Autodesk Inventor part; units mm, degrees
ref_plane "YZ Plane" through (0, 0, 0) normal (1, 0, 0) x (0, 1, 0)
ref_plane "XZ Plane" through (0, 0, 0) normal (0, 1, 0) x (-1, 0, 0)
ref_plane "XY Plane" through (0, 0, 0) normal (0, 0, 1) x (1, 0, 0)
sketch "Esquisse1" plane through (0, 0, 0) normal (0, 1, 0) x (-1, 0, 0)
  line L0 (20.5, 10.5) -> (-20.5, 10.5)
  line L1 (-20.5, 10.5) -> (-20.5, -10.5)
  line L2 (-20.5, -10.5) -> (20.5, -10.5)
  line L3 (20.5, -10.5) -> (20.5, 10.5)
  line L4 (28.5, 12.5) -> (-36.5, 12.5)
  line L5 (-36.5, 12.5) -> (-36.5, -12.5)
  line L6 (-36.5, -12.5) -> (28.5, -12.5)
  line L7 (28.5, -12.5) -> (28.5, 12.5)
  line L8 (-36.5, -12.5) -> (-45.5993, 12.5)
  line L9 (-45.5993, 12.5) -> (-36.5, 12.5)
  point P0 (0, 0)
  dimension "d0" = 20
  dimension "d1" = 41
  dimension "d2" = 21
  dimension "d3" = 10.5
  dimension "d4" = 20.5
  dimension "d5" = 8
  dimension "d6" = 2
  dimension "d7" = 2
  dimension "d8" = 16
extrude "Extrusion1" add sketch "Esquisse1" along normal mid plane 25
sketch "Esquisse2" plane through (36.5, -12.5, -12.5) normal (0.9397, 0, -0.342) x (-0.342, 0, -0.9397)
  line L0 (-26.6044, 25) -> (0, 0)
  line L1 (0, 0) -> (0, 25)
  line L2 (0, 25) -> (-26.6044, 0)
  arc A0 (-8.3022, 22.298) -> (-18.3022, 22.298) centre (-13.3022, 12.5) ccw
  line L3 (-18.3022, 22.298) -> (-8.3022, 22.298)
  line L4 (-8.3022, 22.298) -> (-8.3022, 2.702)
  line L5 (-8.3022, 2.702) -> (-18.3022, 2.702)
  line L6 (-18.3022, 2.702) -> (-18.3022, 22.298)
  arc A1 (-8.3022, 2.702) -> (-8.3022, 22.298) centre (-13.3022, 12.5) ccw
  arc A2 (-18.3022, 2.702) -> (-8.3022, 2.702) centre (-13.3022, 12.5) ccw
  arc A3 (-18.3022, 22.298) -> (-18.3022, 2.702) centre (-13.3022, 12.5) ccw
  point P0 (0.7376, 12.5)
  dimension "d11" = 22
  dimension "d13" = 10
extrude "Extrusion2" add sketch "Esquisse2" along normal blind 5 contours A3 L6 L0 | L0 L6 L2 A3 | L6 L3 L4 L2 L0 | L0 L2 L6 | L2 L6 A3 | L2 L4 L0 | L0 L4 L5 L6 L2 | A1 L2 L4 | L4 L2 A1 L0 | L0 A1 L4
sketch "Esquisse3" plane through (39.3395, -9.798, -4.6985) normal (0, -1, 0) x (0.9397, 0, -0.342)
  line L0 (5, 10) -> (0, 0)
  line L1 (0, 10) -> (5, 0)
  circle A0 centre (2.5, 5) radius 1.75
  point P0 (-38.574, -9.0398)
  dimension "d16" = 3.5
extrude "Extrusion3" cut sketch "Esquisse3" against normal through all
sketch "Esquisse4" plane through (20.5, -12.5, 10.5) normal (-1, 0, 0) x (0, 0, 1)
  line L0 (-21, 3) -> (0, 3)
  line L1 (0, 3) -> (0, 6)
  line L2 (0, 6) -> (-21, 6)
  line L3 (-21, 6) -> (-21, 3)
  line L4 (-21, 0) -> (-21, 25)
  line L5 (0, 0) -> (0, 25)
  line L6 (0, 0) -> (-21, 0)
  point P0 (-10.5, 12.5)
  dimension "d19" = 3
  dimension "d20" = 3
extrude "Extrusion4" cut sketch "Esquisse4" against normal blind 7 contours L3 L2 L1 L0
sketch "Esquisse5" plane through (-20.5, -12.5, -10.5) normal (1, 0, 0) x (0, 0, -1)
  line L0 (-21, 6) -> (0, 6)
  line L1 (0, 6) -> (0, 3)
  line L2 (0, 3) -> (-21, 3)
  line L3 (-21, 3) -> (-21, 6)
  line L4 (-21, 25) -> (-21, 0)
  line L5 (0, 0) -> (0, 25)
  line L6 (0, 0) -> (-21, 0)
  point P0 (-10.5, 12.5)
  dimension "d23" = 3
  dimension "d24" = 3
extrude "Extrusion5" cut sketch "Esquisse5" against normal blind 7 contours L0 L1 L2 L3
sketch "Esquisse6" plane through (20.5, 12.5, -10.5) normal (-1, 0, 0) x (0, 0, 1)
  line L0 (21, -25) -> (0, 0)
  line L1 (0, -25) -> (21, 0)
  circle A0 centre (10.5, -12.5) radius 4
  dimension "d27" = 8
extrude "Extrusion6" cut sketch "Esquisse6" against normal through all
sketch "Esquisse7" plane through (20.5, 12.5, -10.5) normal (-1, 0, 0) x (0, 0, 1)
  circle A0 centre (10.5, -12.5) radius 4
  circle A1 centre (10.5, -12.5) radius 1.75
  circle A2 centre (10.5, -12.5) radius 4
  dimension "d30" = 0
  dimension "d31" = 3.5
extrude "Extrusion7" add sketch "Esquisse7" against normal blind 18
sketch "Esquisse8" plane through (20.5, 12.5, -10.5) normal (-1, 0, 0) x (0, 0, 1)
  circle A0 centre (10.5, -12.5) radius 3
  dimension "d34" = 6
extrude "Extrusion8" cut sketch "Esquisse8" against normal blind 3
sketch "Esquisse10" plane through (0, -12.5, 0) normal (0, -1, 0) x (1, 0, 0)
  line L0 (-20.5, -10.5) -> (-27.5, -10.5)
  line L1 (-27.5, -10.5) -> (-27.5, 10.5)
  line L2 (-27.5, 10.5) -> (-20.5, 10.5)
  line L3 (-20.5, 10.5) -> (-20.5, -10.5)
  line L4 (20.5, -10.5) -> (27.5, -10.5)
  line L5 (27.5, -10.5) -> (27.5, 10.5)
  line L6 (27.5, 10.5) -> (20.5, 10.5)
  line L7 (20.5, 10.5) -> (20.5, -10.5)
  line L8 (-27.5, -10.5) -> (-27.5, 10.5)
  line L9 (27.5, 10.5) -> (27.5, -10.5)
  line L10 (-27.5, -10.5) -> (-20.5, 0)
  line L11 (-20.5, 0) -> (-27.5, 10.5)
  line L12 (-27.5, 0) -> (-20.5, 10.5)
  line L13 (-20.5, -10.5) -> (-27.5, 0)
  line L14 (20.5, -10.5) -> (27.5, 0)
  line L15 (20.5, 0) -> (27.5, -10.5)
  line L16 (27.5, 10.5) -> (20.5, 0)
  line L17 (20.5, 10.5) -> (27.5, 0)
  circle A0 centre (-24, -5.25) radius 2
  circle A1 centre (24, -5.25) radius 2
  circle A2 centre (24, 5.25) radius 2
  circle A3 centre (-24, 5.25) radius 2
  point P0 (0, 0)
  dimension "d37" = 4
  dimension "d38" = 4
  dimension "d39" = 4
  dimension "d40" = 4
extrude "Extrusion9" cut sketch "Esquisse10" against normal through all contours A0 L10 L13 | L13 L10 A0 | A0 L13 L10 | L10 L13 A0 | A3 L12 L11 | L11 L12 A3 | A3 L11 L12 | L12 L11 A3 | A1 L15 L14 | L14 L15 A1 | L15 L14 A1 | A1 L14 L15 | A2 L17 L16 | L16 L17 A2 | L17 L16 A2 | A2 L16 L17
sketch "Esquisse11" plane through (36.5, 12.5, -12.5) normal (0, 0, -1) x (-1, 0, 0)
  line L0 (65, 0) -> (45, 0)
  line L1 (45, 0) -> (45, -13)
  line L2 (45, -13) -> (65, -13)
  line L3 (65, -13) -> (65, 0)
  line L4 (65, -25) -> (0, -25)
  line L5 (45, -13) -> (32, 0)
  line L6 (0, 0) -> (65, 0)
  line L7 (45, 0) -> (32, 0)
  point P0 (36.5, -12.5)
  dimension "d43" = 20
  dimension "d44" = 12
  dimension "d45" = 45
extrude "Extrusion10" cut sketch "Esquisse11" against normal through all
sketch "Esquisse12" plane through (-28.5, -12.5, 12.5) normal (0, 0, 1) x (1, 0, 0)
  line L0 (33, 25) -> (74.0993, 25)
  line L1 (74.0993, 0) -> (60.5, 0)
  line L2 (60.5, 0) -> (60.5, 25)
  line L3 (60.5, 25) -> (74.0993, 25)
  line L4 (74.0993, 25) -> (74.0993, 0)
  line L5 (56, 6) -> (56, 3)
  line L6 (65, 25) -> (65, 0)
  line L7 (60.5, 25) -> (0, 25)
  line L8 (0, 25) -> (0, 0)
  line L9 (0, 0) -> (60.5, 0)
  line L10 (60.5, 0) -> (60.5, 25)
  point P0 (28.5, 12.5)
  dimension "d48" = 9
  dimension "d49" = 4.5
extrude "Extrusion11" cut sketch "Esquisse12" against normal through all contours L0 L2 L9 L8 L7
equation "\"d38\" = d37"
equation "\"d39\" = d37"
equation "\"d40\" = d37"
equation "\"d49\" = 0.5 * d48"
properties part number "forearm"
Geometry check sheet. Reference: the model listing, model coordinates, mm. A direction names the side the tool comes from. Coordinates: 2 decimals unless noted, no trailing zeros. Order: outer loops, then holes, each group sorted by start corner. A loop starts at its lowest first (then second) coordinate and runs counter-clockwise, first axis right, second up. Notation, with made-up numbers: (-11, 18.5) -> (-7, 18.5) arc R20 cw to (-7, 29.5) -> close; hole circle Ø10 at (-28, 42.25). An arc over 180 degrees is marked (long way). Use a Markdown table: item, result. Add a question column.
1. Cross-section at A-A (x = 34). Enter the section's corners in (y, z).
2. Cross-section at D-D (y = 8.25). Enter the section's corners in (x, z), and give its area (3 significant figures).
3. Go/stop test with flat-tipped pins: pin 1 Ø4 at (x, z) = (43.4, -0.86) entering from -Y; pin 2 Ø1 at (x, z) = (46, 2.5) entering from +Y; pin 3 Ø7 at (y, z) = (0, 0) entering from +X. Record where each tip stops, or that it passes through.
4. Cross-section at C-C (y = 0). Enter the section's corners in (x, z), and give its area (3 significant figures).
5. Cross-section at B-B (z = 0). Enter the section's corners in (x, y), and give its area (3 significant figures).
6. Mould release check, pull along X, two halves, no side actions. Record for faces 5 (the face through (41, 9.798, -1)), 6 (the face through (38.5, -2, 1)), 7 (the face through (42.46, 6.37, -2.33)), 8 (the face through (43.63, -6.46, -2.59)): pulls with the +X half, pulls with the -X half, needs draft (parallel to the pull), parting line crosses it, or undercut.
7. Material ranges on L1, parallel to Y at x = 34.25, z = 0; L2, parallel to Y at x = 40.5, z = 0; L3, parallel to X at y = -3.5, z = -2, recorded low to high.
8. Set-up check for faces 1 (the face through (39.604, 0.169, -11.179)), 2 (the face through (42.062, -1.532, 3.695)), 3 (the face through (32, 0, 3)), 4 (the face through (41, -9.798, -1)): record each of +Z, -Z, +X, -X, +Y, -Y from which the full face is reachable in a straight line by a thin tool's end or side.
Filled sheet:
| question | item | result |
|---|---|---|
| 1 | outline | (-12.5, -12.5) -> (12.5, -12.5) -> (12.5, 12.5) -> (-12.5, 12.5) -> close; hole circle Ø3.5 at (0, 0) |
| 2 | outline | (32, -12.5) -> (36.5, -12.5) -> (38.56, -6.84) -> (43.26, -8.55) -> (48.24, 5.13) -> (43.54, 6.84) -> (45.6, 12.5) -> (32, 12.5) -> close; hole circle Ø3.5 at (43.4, -0.86) |
| 2 | area | 289 mm2 |
| 3 | pin 1 | y = -9.8 |
| 3 | pin 2 | y = 9.8 |
| 3 | pin 3 | x = 38.5 |
| 4 | outline | (32, -12.5) -> (36.5, -12.5) -> (37.29, -10.34) -> (41.99, -12.05) -> (44.91, -4) -> (38.5, -4) -> (38.5, -1.75) -> (32, -1.75) -> close; (32, 1.75) -> (38.5, 1.75) -> (38.5, 4) -> (47.83, 4) -> (49.51, 8.63) -> (44.81, 10.34) -> (45.6, 12.5) -> (32, 12.5) -> close |
| 4 | area | 251 mm2 |
| 5 | outline | (32, -12.5) -> (41.05, -12.5) -> (41.05, -9.8) -> (41.87, -9.8) -> (41.87, -4) -> (38.5, -4) -> (38.5, -1.75) -> (32, -1.75) -> close; (32, 1.75) -> (38.5, 1.75) -> (38.5, 4) -> (41.87, 4) -> (41.87, 9.8) -> (41.05, 9.8) -> (41.05, 12.5) -> (32, 12.5) -> close; (44.93, -9.8) -> (46.37, -9.8) -> (46.37, -4) -> (44.93, -4) -> close; (44.93, 4) -> (46.37, 4) -> (46.37, 9.8) -> (44.93, 9.8) -> close |
| 5 | area | 209 mm2 |
| 6 | face 5 | needs draft |
| 6 | face 6 | pulls with the +X half |
| 6 | face 7 | undercut |
| 6 | face 8 | undercut |
| 7 | L1 | -12.5 to -1.75, 1.75 to 12.5 |
| 7 | L2 | -12.5 to -4, 4 to 12.5 |
| 7 | L3 | 32 to 42.08, 44.72 to 45.64 |
| 8 | face 1 | -Z |
| 8 | face 2 | +X |
| 8 | face 3 | +Z, -Z, -X, +Y, -Y |
| 8 | face 4 | -Z, +X, -Y |
